```python
from build123d import *

# Parameters (mm, degrees)
BOSS_EXTRU_1_DEPTH        = 5
BOSS_EXTRU_1_DEPTH_BACK   = 10
ESQUISSE1_R               = 1.75
BOSS_EXTRU_1_2_DEPTH      = 5
BOSS_EXTRU_1_2_DEPTH_BACK = 10
ESQUISSE2_R               = 1.75
ESQUISSE3_R               = 1.75
ENL_V_MAT_EXTRU_1_DEPTH   = 3
ESQUISSE4_R               = 1.75
ESQUISSE5_R               = 1.75
ENL_V_MAT_EXTRU_2_DEPTH   = 3


with BuildPart() as part:
    # Esquisse1 → Boss.-Extru.1 (new, two sides: drawn at the far end of the back side and taken through both)
    with BuildSketch(Plane.XY.offset(-BOSS_EXTRU_1_DEPTH_BACK)):
        with Locations((-1.8, 0)):
            Circle(ESQUISSE1_R)
    extrude(amount=BOSS_EXTRU_1_DEPTH + BOSS_EXTRU_1_DEPTH_BACK)



with BuildPart() as body_2:
    # Esquisse1 → Boss.-Extru.1 2 (new, two sides: drawn at the far end of the back side and taken through both)
    with BuildSketch(Plane.XY.offset(-BOSS_EXTRU_1_2_DEPTH_BACK)):
        with Locations((1.8, 0)):
            Circle(ESQUISSE1_R)
    extrude(amount=BOSS_EXTRU_1_2_DEPTH + BOSS_EXTRU_1_2_DEPTH_BACK)

    # Balayage1: sweep along a curve in space
    with BuildLine() as balayage1_path:
        Line((1.8, 0, 5.5), (1.8, 0, 5))
        ThreePointArc((-0.050422137, 0, 9.833705523), (1.318037114, 0, 7.856112563), (1.8, 0, 5.5))
        Line((-0.050422137, 0, 9.833705523), (-5.259213711, 0, 14.821189351))
        ThreePointArc((-4.816825334, 0.348555806, 18.022401208), (-5.861081542, 0.11010529, 16.542524811), (-5.259213711, 0, 14.821189351))
        Line((-4.816825334, 0.348555806, 18.022401208), (-4.769816548, 0.355226106, 18.046757443))
        ThreePointArc((-2.772717213, 0.5, 17.953095794), (-3.761180865, 0.461194336, 18.266892532), (-4.769816548, 0.355226106, 18.046757443))
        Line((6.371171623, 0.5, 12.127796149), (-2.772717213, 0.5, 17.953095794))
    # Esquisse2 → Balayage1 (sweep)
    with BuildSketch(Plane.XY.offset(5)):
        with Locations((1.8, 0)):
            Circle(ESQUISSE2_R)
    sweep(path=balayage1_path.line)

    # Esquisse3 → Enlèv. mat.-Extru.1 (cut)
    with BuildSketch(Plane(origin=(-0.963885494, 0, 0.614062783), x_dir=(-0.5372996083468307, 1.153766929709301e-15, -0.8433914458128813), z_dir=(0.8433914458128813, -1.8110513089197862e-15, -0.5372996083468307))):
        with Locations((-13.651707546, 0.5)):
            Circle(ESQUISSE3_R)
    extrude(amount=-ENL_V_MAT_EXTRU_1_DEPTH, mode=Mode.SUBTRACT)


with BuildPart() as part_1:
    add(part.part)

    add(body_2.part)  # Balayage2 merges body 2
    # Balayage2: sweep along a curve in space
    with BuildLine() as balayage2_path:
        Line((-1.8, 0, 5), (-1.8, 0, 5.5))
        ThreePointArc((-3.277669531, 0, 8.085055114), (-2.195485515, 0, 6.988792899), (-1.8, 0, 5.5))
        Line((-3.277669531, 0, 8.085055114), (-9.10744265, 0, 11.518189362))
        ThreePointArc((-13.19492784, 0.134768754, 16.117942999), (-11.513609411, 0.034530095, 13.496967314), (-9.10744265, 0, 11.518189362))
        Line((-14.679034762, 0.288575292, 19.494314724), (-13.19492784, 0.134768754, 16.117942999))
        ThreePointArc((-21.673024109, 0.5, 25.233780857), (-17.489247519, 0.444119723, 23.199109722), (-14.679034762, 0.288575292, 19.494314724))
        Line((-29.410957851, 0.5, 26.949239467), (-21.673024109, 0.5, 25.233780857))
    # Esquisse4 → Balayage2 (sweep)
    with BuildSketch(Plane.XY.offset(5)):
        with Locations((-1.8, 0)):
            Circle(ESQUISSE4_R)
    sweep(path=balayage2_path.line)

    # Esquisse5 → Enlèv. mat.-Extru.2 (cut)
    with BuildSketch(Plane(origin=(-33.727789357, 0, 7.477270883), x_dir=(0.21643961393810765, 0, 0.9762960071199323), z_dir=(-0.9762960071199324, 0, 0.21643961393810768))):
        with Locations((19.944738524, 0.5)):
            Circle(ESQUISSE5_R)
    extrude(amount=-ENL_V_MAT_EXTRU_2_DEPTH, mode=Mode.SUBTRACT)


solid = part_1.part
```
Can you work these out from the model? Positions are in its coordinate system, mm. A direction names the side the tool comes from. Give positions to 0.01 mm unless a question says otherwise; leave off trailing zeros. Order: outer loops, then holes, each group sorted by start corner. A loop starts at its lowest first (then second) coordinate and runs counter-clockwise, first axis right, second up. Notation, with made-up numbers: M -31.5,-18.75 L 26.5,-18.75 A16 ccw 26.5,-6.75 Z; hole C 30,62.5 d1. An arc over 180 degrees is marked long. One line per item, written item: value.
1) I want a section at B-B, the plane x = -3. Count the separate pieces of the cut face and the enclosed holes in it, plus the area to 3 significant figures.
Answer sheet:
separate pieces: 3
enclosed holes: 0
area: 76.5 mm^2
2) On a 3-axis mill with a long thin cutter (end or side, diameter ignored), from which of +Z, -Z, +X, -X, +Y, -Y can I reach the whole of each face in a straight line? I mean faces 1 (the face through (3.854, 0.524, 13.76)), 2 (the face through (-2, 0, -10)). Say none if no direction works.
Answer sheet:
face 1: +X, +Y, -Y
face 2: -Z, +X, -X, +Y, -Y
3) Please list where these lines run through material, in increasing order: line 1 along Z through (x, y) = (-4, -0.45); line 2 along X through (y, z) = (-0.55, 13); line 3 along X through (y, z) = (0.3, 13.5).
Answer sheet:
line 1: z = 6.54 to 10.47, 11.27 to 15.96, 16.7 to 19.77
line 2: x = -13.24 to -8.35, -5.76 to -0.96, 2.4 to 3.37
line 3: x = -13.71 to -8.98, -6.37 to -1.39, 0.98 to 3.69
4) We'd pull the mould along Z, two halves only. Please class faces 3 (the face through (2, 0, -10)), 4 (the face through (-12.487, -0.479, 18.503)), 5 (the face through (-1.464, -0.526, 13.498)), 6 (the face through (-26.487, 0.524, 26.276)): released by +Z, released by -Z, zero draft, split by the parting line, or undercut.
Answer sheet:
face 3: released by -Z
face 4: split by the parting line
face 5: undercut
face 6: released by +Z
5) For P1, Ø6, axis at x = -5.5, z = 11, coming from the -Y side, with a flat end and sliding along its axis, tell me the tip position at first contact or that it passes through.
Answer sheet:
P1: stops at y = -1.75
6) I want a section at A-A, the plane z = -1.5. List the corners of the cut face in (x, y) for me, plus the area to 3 significant figures.
Answer sheet:
outline: C -1.8,0 d3.5; C 1.8,0 d3.5
area: 19.2 mm^2
